from build123d import *

# Parameters (mm, degrees)
SKETCH1_W           = 10
SKETCH1_H           = 10
BOSS_EXTRUDE1_DEPTH = 17
CUT_EXTRUDE1_DEPTH  = 17


with BuildPart() as part:
    # Sketch1 → Boss-Extrude1 (new body)
    with BuildSketch(Plane(origin=(0, 0, 0), x_dir=(1, 0, 0), z_dir=(0, 1, 0))):
        with Locations((5, 5)):
            Rectangle(SKETCH1_W, SKETCH1_H)
    extrude(amount=BOSS_EXTRUDE1_DEPTH)

    # Sketch2 → Cut-Extrude1 (cut)
    with BuildSketch(Plane(origin=(0, 17, 0), x_dir=(1, 0, 0), z_dir=(0, 1, 0))):
        with BuildLine():
            ThreePointArc((7.61629509, 7.61629509), (2.38370491, 7.61629509), (2.38370491, 2.38370491))
            Line((2.38370491, 2.38370491), (7.61629509, 7.61629509))
        make_face()
        with BuildLine():
            Line((7.61629509, 7.61629509), (2.38370491, 2.38370491))
            ThreePointArc((2.38370491, 2.38370491), (6.4159287, 1.58164573), (8.7, 5))
            ThreePointArc((8.7, 5), (8.41835427, 6.4159287), (7.61629509, 7.61629509))
        make_face()
    extrude(amount=-CUT_EXTRUDE1_DEPTH, mode=Mode.SUBTRACT)


solid = part.part
The model under review builds one solid part; all positions refer to its coordinate system, in mm. Round coordinates to 2 decimals unless told otherwise and drop trailing zeros. Loops run counter-clockwise (first coordinate to the right, second up) from the corner with the lowest first, then second, coordinate; pieces in that order, holes last. Notation, with made-up numbers: (-5.75, 6.25) -> (2.25, 6.25) arc R31 cw to (2.25, 39.25) -> close; hole circle Ø10 at (-18.5, 35.5). An arc over 180 degrees is marked (long way). Write item = value, one per line. Start each with the question number.
Item 1: Take a section at A-A on y = 9.25. Give the boundary of the cut face in (x, z), plus the area to 3 significant figures.
Item 2: To check wall thickness, follow L1, parallel to Z at x = 8.25, y = 3; L2, parallel to Z at x = 6.75, y = 11.25; L3, parallel to X at y = 14.5, z = -6.5. State the ranges of each line that lie inside material, in increasing order.
Item 3: Insertion check: pin 1 (1.5 mm diameter, centred on x = 5.5, z = -4, fed in from +Y). The pin has a flat end and moves straight along its axis. Give the tip position at first contact, or say it passes through.
Item 4: Take a section at B-B on x = 5. Give the boundary of the cut face in (y, z).
Item 5: Take a section at C-C on z = -5.25. Give the boundary of the cut face in (x, y), plus the area to 3 significant figures.
Result:
q1.outline = (0, -10) -> (10, -10) -> (10, 0) -> (0, 0) -> close; hole circle Ø7.4 at (5, -5)
q1.area = 57.0 mm²
q2.L1 = -10 to -6.77, -3.23 to 0
q2.L2 = -10 to -8.26, -1.74 to 0
q2.L3 = 0 to 1.62, 8.38 to 10
q3.pin_1 = through
q4.outline = (0, -10) -> (17, -10) -> (17, -8.7) -> (0, -8.7) -> close; (0, -1.3) -> (17, -1.3) -> (17, 0) -> (0, 0) -> close
q5.outline = (0, 0) -> (1.31, 0) -> (1.31, 17) -> (0, 17) -> close; (8.69, 0) -> (10, 0) -> (10, 17) -> (8.69, 17) -> close
q5.area = 44.5 mm²
